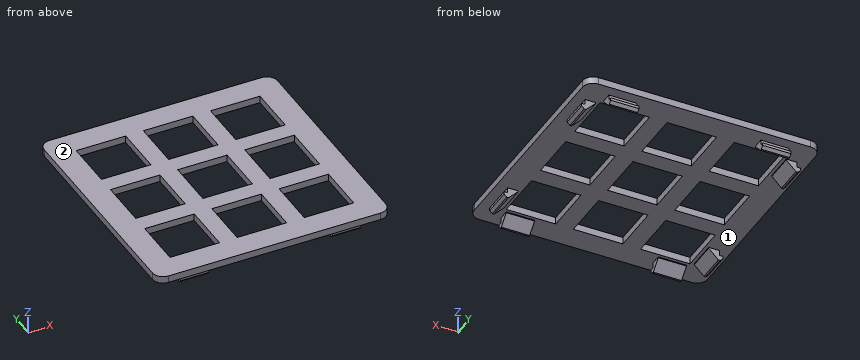
from build123d import *

# Parameters (mm, degrees)
SKETCH_W        = 14
SKETCH_H        = 14
PAD_DEPTH       = 2
SKETCH004_W     = 8
SKETCH004_H     = 3
SKETCH004_W_2   = 3
SKETCH004_H_2   = 8
PAD003_DEPTH    = 3
SKETCH005_W     = 8
SKETCH005_H     = 1.5
PAD004_DEPTH    = 1
SKETCH008_W     = 8
SKETCH008_H     = 1.5
PAD005_DEPTH    = 1
SKETCH007_W     = 8
SKETCH007_H     = 1.5
PAD006_DEPTH    = 1
SKETCH006_W     = 8
SKETCH006_H     = 1.5
PAD007_DEPTH    = 1
CHAMFER_SIZE    = 2.75
CHAMFER001_SIZE = 0.75


with BuildPart() as part:
    # Sketch → Pad (new body)
    with BuildSketch(Plane.XY):
        with BuildLine():
            Line((-30, 33), (30, 33))
            ThreePointArc((33, 30), (32.12132, 32.12132), (30, 33))
            Line((33, 30), (33, -30))
            ThreePointArc((30, -33), (32.12132, -32.12132), (33, -30))
            Line((30, -33), (-30, -33))
            ThreePointArc((-33, -30), (-32.12132, -32.12132), (-30, -33))
            Line((-33, -30), (-33, 30))
            ThreePointArc((-30, 33), (-32.12132, 32.12132), (-33, 30))
        make_face()
        Rectangle(SKETCH_W, SKETCH_H, mode=Mode.SUBTRACT)
        with Locations((19, 0)):
            Rectangle(SKETCH_W, SKETCH_H, mode=Mode.SUBTRACT)
        with Locations((-19, 0)):
            Rectangle(SKETCH_W, SKETCH_H, mode=Mode.SUBTRACT)
        with Locations((0, 19)):
            Rectangle(SKETCH_W, SKETCH_H, mode=Mode.SUBTRACT)
        with Locations((19, 19)):
            Rectangle(SKETCH_W, SKETCH_H, mode=Mode.SUBTRACT)
        with Locations((-19, 19)):
            Rectangle(SKETCH_W, SKETCH_H, mode=Mode.SUBTRACT)
        with Locations((0, -19)):
            Rectangle(SKETCH_W, SKETCH_H, mode=Mode.SUBTRACT)
        with Locations((19, -19)):
            Rectangle(SKETCH_W, SKETCH_H, mode=Mode.SUBTRACT)
        with Locations((-19, -19)):
            Rectangle(SKETCH_W, SKETCH_H, mode=Mode.SUBTRACT)
    extrude(amount=PAD_DEPTH)

    # Sketch004 (on DatumPlane) → Pad003 (join)
    with BuildSketch(Plane(origin=(0, 0, 0), x_dir=(1, 0, 0), z_dir=(0, 0, -1))):
        with Locations((-21.5, -28.45)):
            Rectangle(SKETCH004_W, SKETCH004_H)
        with Locations((-28.45, -21.5)):
            Rectangle(SKETCH004_W_2, SKETCH004_H_2)
        with Locations((21.5, -28.45)):
            Rectangle(SKETCH004_W, SKETCH004_H)
        with Locations((28.45, -21.5)):
            Rectangle(SKETCH004_W_2, SKETCH004_H_2)
        with Locations((-28.45, 21.5)):
            Rectangle(SKETCH004_W_2, SKETCH004_H_2)
        with Locations((28.45, 21.5)):
            Rectangle(SKETCH004_W_2, SKETCH004_H_2)
        with Locations((-21.5, 28.45)):
            Rectangle(SKETCH004_W, SKETCH004_H)
        with Locations((21.5, 28.45)):
            Rectangle(SKETCH004_W, SKETCH004_H)
    extrude(amount=PAD003_DEPTH)

    # Sketch005 (on Face43 of Pad003) → Pad004 (join)
    with BuildSketch(Plane.YZ.offset(29.95)):
        with Locations((-21.5, -2.25)):
            Rectangle(SKETCH005_W, SKETCH005_H)
        with Locations((21.5, -2.25)):
            Rectangle(SKETCH005_W, SKETCH005_H)
    extrude(amount=PAD004_DEPTH)

    # Sketch008 (on Face11 of Pad003) → Pad005 (join)
    with BuildSketch(Plane.XZ.offset(29.95)):
        with Locations((-21.5, -2.25)):
            Rectangle(SKETCH008_W, SKETCH008_H)
        with Locations((21.5, -2.25)):
            Rectangle(SKETCH008_W, SKETCH008_H)
    extrude(amount=PAD005_DEPTH)

    # Sketch007 (on Face51 of Pad003) → Pad006 (join)
    with BuildSketch(Plane(origin=(-29.95, 0, 0), x_dir=(0, -1, 0), z_dir=(-1, 0, 0))):
        with Locations((-21.5, -2.25)):
            Rectangle(SKETCH007_W, SKETCH007_H)
        with Locations((21.5, -2.25)):
            Rectangle(SKETCH007_W, SKETCH007_H)
    extrude(amount=PAD006_DEPTH)

    # Sketch006 (on Face75 of Pad003) → Pad007 (join)
    with BuildSketch(Plane(origin=(0, 29.95, 0), x_dir=(-1, 0, 0), z_dir=(0, 1, 0))):
        with Locations((-21.5, -2.25)):
            Rectangle(SKETCH006_W, SKETCH006_H)
        with Locations((21.5, -2.25)):
            Rectangle(SKETCH006_W, SKETCH006_H)
    extrude(amount=PAD007_DEPTH)

    # Chamfer
    chamfer_edges = [part.edges().sort_by_distance(p)[0] for p in [
        (-26.95, -21.5, -3),
        (-21.5, -26.95, -3),
        (21.5, -26.95, -3),
        (26.95, -21.5, -3),
        (-26.95, 21.5, -3),
        (-21.5, 26.95, -3),
        (21.5, 26.95, -3),
        (26.95, 21.5, -3),
    ]]
    chamfer(chamfer_edges, length=CHAMFER_SIZE)

    # Chamfer001
    chamfer001_edges = [part.edges().sort_by_distance(p)[0] for p in [
        (30.95, 21.5, -3),
        (21.5, 30.95, -3),
        (-21.5, 30.95, -3),
        (-30.95, 21.5, -3),
        (-30.95, -21.5, -3),
        (-21.5, -30.95, -3),
        (21.5, -30.95, -3),
        (30.95, -21.5, -3),
    ]]
    chamfer(chamfer001_edges, length=CHAMFER001_SIZE)


solid = part.part
Verification items for the finished model (mm, model axes). Face numbers are marked on the shaded views. Round coordinates to 2 decimals unless told otherwise and drop trailing zeros. Write each loop counter-clockwise with the first axis right and the second up, starting at its lowest first coordinate (ties: lowest second). Pieces come first, ordered by that corner, then holes.
(1) Depth check by flat-ended pin: pin 1 Ø0.8 at (x, z) = (-23.5, -2) entering from +Y; pin 2 Ø4 at (x, y) = (-20, 4) entering from +Z; pin 3 Ø3 at (y, z) = (18.5, -2.5) entering from -X; pin 4 Ø5 at (x, y) = (-5, 17) entering from -Z. Enter the tip coordinate at first touch or a pass-through.
Returned:
pin 1: stops at y = 30.95
pin 2: passes through
pin 3: stops at x = -30.95
pin 4: stops at z = 0
(2) Material ranges on line 1 (X direction, y = -13, z = 0.15); line 2 (Y direction, x = 24.5, z = -0.2), recorded low to high.
Returned:
line 1: x = -33 to -26, -12 to -7, 7 to 12, 26 to 33
line 2: y = -29.95 to -26.95, 26.95 to 29.95
(3) Mould release check, pull along X, two halves, no side actions. Record for the marked faces 1 and 2: pulls with the +X half, pulls with the -X half, needs draft (parallel to the pull), parting line crosses it, or undercut.
Returned:
face 1: undercut
face 2: needs draft
(4) Section check A-A (y = -19). Give the number of separate pieces and of enclosed holes in the cut face, plus the area to 3 significant figures.
Returned:
separate pieces: 4
enclosed holes: 0
area: 60.9 mm2
(5) Section check C-C (y = 4). Enter the section's corners in (x, z).
Returned:
outline: (-33, 0) - (-26, 0) - (-26, 2) - (-33, 2) - close; (-12, 0) - (-7, 0) - (-7, 2) - (-12, 2) - close; (7, 0) - (12, 0) - (12, 2) - (7, 2) - close; (26, 0) - (33, 0) - (33, 2) - (26, 2) - close
